```python
from build123d import *

# Parameters (mm, degrees)
EXTRUDE1_DEPTH          = 49.784
EXTRUDE1_DEPTH_BACK     = 49.784
SKETCH1_R               = 19.05
EXTRUDE2_DEPTH          = 49.784
EXTRUDE2_DEPTH_BACK     = 49.784
SKETCH2_R               = 19.05
EXTRUDE3_DEPTH          = 49.784
EXTRUDE3_DEPTH_BACK     = 49.784
SKETCH3_R               = 19.05
CUT_EXTRUDE1_DEPTH      = 87.228417404
CUT_EXTRUDE1_DEPTH_BACK = 87.228417404
SKETCH4_R               = 17.399
CUT_EXTRUDE2_DEPTH      = 87.228417404
CUT_EXTRUDE2_DEPTH_BACK = 87.228417404
SKETCH5_R               = 17.399
CUT_EXTRUDE3_DEPTH      = 87.228417404
CUT_EXTRUDE3_DEPTH_BACK = 87.228417404
SKETCH6_R               = 17.399


with BuildPart() as part:
    # Sketch1 → Extrude1 (new, two sides: drawn at the far end of the back side and taken through both)
    with BuildSketch(Plane(origin=(0, 0, 0), x_dir=(1, 0, 0), z_dir=(0, 1, 0)).offset(-EXTRUDE1_DEPTH_BACK)):
        with Locations(Location((0, 0, 0), (0, 0, 270))):
            Circle(SKETCH1_R)
    extrude(amount=EXTRUDE1_DEPTH + EXTRUDE1_DEPTH_BACK)

    # Sketch2 → Extrude2 (add, two sides: drawn at the far end of the back side and taken through both)
    with BuildSketch(Plane.XY.offset(-EXTRUDE2_DEPTH_BACK)):
        Circle(SKETCH2_R)
    extrude(amount=EXTRUDE2_DEPTH + EXTRUDE2_DEPTH_BACK)

    # Sketch3 → Extrude3 (add, two sides: drawn at the far end of the back side and taken through both)
    with BuildSketch(Plane(origin=(0, 0, 0), x_dir=(0, 0, -1), z_dir=(1, 0, 0)).offset(-EXTRUDE3_DEPTH_BACK)):
        Circle(SKETCH3_R)
    extrude(amount=EXTRUDE3_DEPTH + EXTRUDE3_DEPTH_BACK)

    # Sketch4 → Cut-Extrude1 (cut, two sides: drawn at the far end of the back side and taken through both)
    with BuildSketch(Plane(origin=(0, 0, 0), x_dir=(1, 0, 0), z_dir=(0, 1, 0)).offset(-CUT_EXTRUDE1_DEPTH_BACK)):
        with Locations(Location((0, 0, 0), (0, 0, 270))):
            Circle(SKETCH4_R)
    extrude(amount=CUT_EXTRUDE1_DEPTH + CUT_EXTRUDE1_DEPTH_BACK, mode=Mode.SUBTRACT)

    # Sketch5 → Cut-Extrude2 (cut, two sides: drawn at the far end of the back side and taken through both)
    with BuildSketch(Plane(origin=(0, 0, 0), x_dir=(0, 0, -1), z_dir=(1, 0, 0)).offset(-CUT_EXTRUDE2_DEPTH_BACK)):
        Circle(SKETCH5_R)
    extrude(amount=CUT_EXTRUDE2_DEPTH + CUT_EXTRUDE2_DEPTH_BACK, mode=Mode.SUBTRACT)

    # Sketch6 → Cut-Extrude3 (cut, two sides: drawn at the far end of the back side and taken through both)
    with BuildSketch(Plane.XY.offset(-CUT_EXTRUDE3_DEPTH_BACK)):
        Circle(SKETCH6_R)
    extrude(amount=CUT_EXTRUDE3_DEPTH + CUT_EXTRUDE3_DEPTH_BACK, mode=Mode.SUBTRACT)


solid = part.part
```
Model file for the job. Use its own axes, mm. A direction names the side the tool comes from. Round coordinates to 2 decimals unless told otherwise and drop trailing zeros. Loops run counter-clockwise (first coordinate to the right, second up) from the corner with the lowest first, then second, coordinate; pieces in that order, holes last. Notation, with made-up numbers: M 43,44 L 90,44 A12 cw 90,65 Z; hole C 37,10 d4. An arc over 180 degrees is marked long. Put each result on its own line as item: value. Start each with the question number.
Item 1: Mould opens along X. For faces 6 (the face through (0.84, 31.37, -19.03)), 7 (the face through (0.77, 30.78, -17.38)), 8 (the face through (-15.43, -49.784, 8.38)) say: released by +X, released by -X, zero draft, split by the parting line, or undercut.
Item 2: Drill centre lines: line 1 along X through (y, z) = (-21, 0); line 2 along Y through (x, z) = (21, -10). Where is each one in solid material? Low to high.
Item 3: Cut at A-A (x = 0). List the corners of the cut face in (y, z).
Item 4: 3-axis set-ups, long thin cutter, end or side, ignore diameter. For faces 1 (the face through (-19.03, 0.84, -31.88)), 2 (the face through (-31.88, 0.84, 19.03)), 3 (the face through (31.37, 0.84, 19.03)), 4 (the face through (-19.03, 0.84, 31.37)), 5 (the face through (0.84, -31.88, -19.03)): which of +Z, -Z, +X, -X, +Y, -Y reach the whole face in a straight line?
Item 5: Cut at C-C (z = -43). List the corners of the cut face in (x, y).
Item 6: Drop flat-ended pins along their axis: P1, Ø3, axis at x = 10, y = 18.5, coming from the -Z side; P2, Ø1.5, axis at x = 16, y = -28, coming from the +Z side; P3, Ø10, axis at y = 4, z = 29.5, coming from the -X side. Give the stop position or say it passes through.
Answer block:
1. face 6: split by the parting line
1. face 7: undercut
1. face 8: zero draft
2. line 1: -19.05 to -17.4, 17.4 to 19.05
2. line 2: -16.21 to -14.24, 14.24 to 16.21
3. outline: M -49.78,-19.05 L -19.05,-19.05 L -19.05,-49.78 L -17.4,-49.78 L -17.4,-17.4 L -49.78,-17.4 Z; M -49.78,17.4 L -17.4,17.4 L -17.4,49.78 L -19.05,49.78 L -19.05,19.05 L -49.78,19.05 Z; M 17.4,-49.78 L 19.05,-49.78 L 19.05,-19.05 L 49.78,-19.05 L 49.78,-17.4 L 17.4,-17.4 Z; M 17.4,17.4 L 49.78,17.4 L 49.78,19.05 L 19.05,19.05 L 19.05,49.78 L 17.4,49.78 Z
4. face 1: -Z
4. face 2: -X
4. face 3: +X
4. face 4: +Z
4. face 5: -Y
5. outline: C 0,0 d38.1; hole C 0,0 d34.8
6. P1: z = -17.05
6. P2: z = 11.42
6. P3: x = -19.05
